Print and shaded views of the part. All mm, measured from the part's lowest x, y and z. A direction names the side the tool comes from. Round coordinates to 2 decimals unless told otherwise and drop trailing zeros. Loops run counter-clockwise (first coordinate to the right, second up) from the corner with the lowest first, then second, coordinate; pieces in that order, holes last. Notation, with made-up numbers: (-33, -14) - (-25, -14) arc R25 ccw to (-25, 2) - close; hole circle Ø11 at (15, 15.25). An arc over 180 degrees is marked (long way). Answer as a JSON object with one key per item and string values.
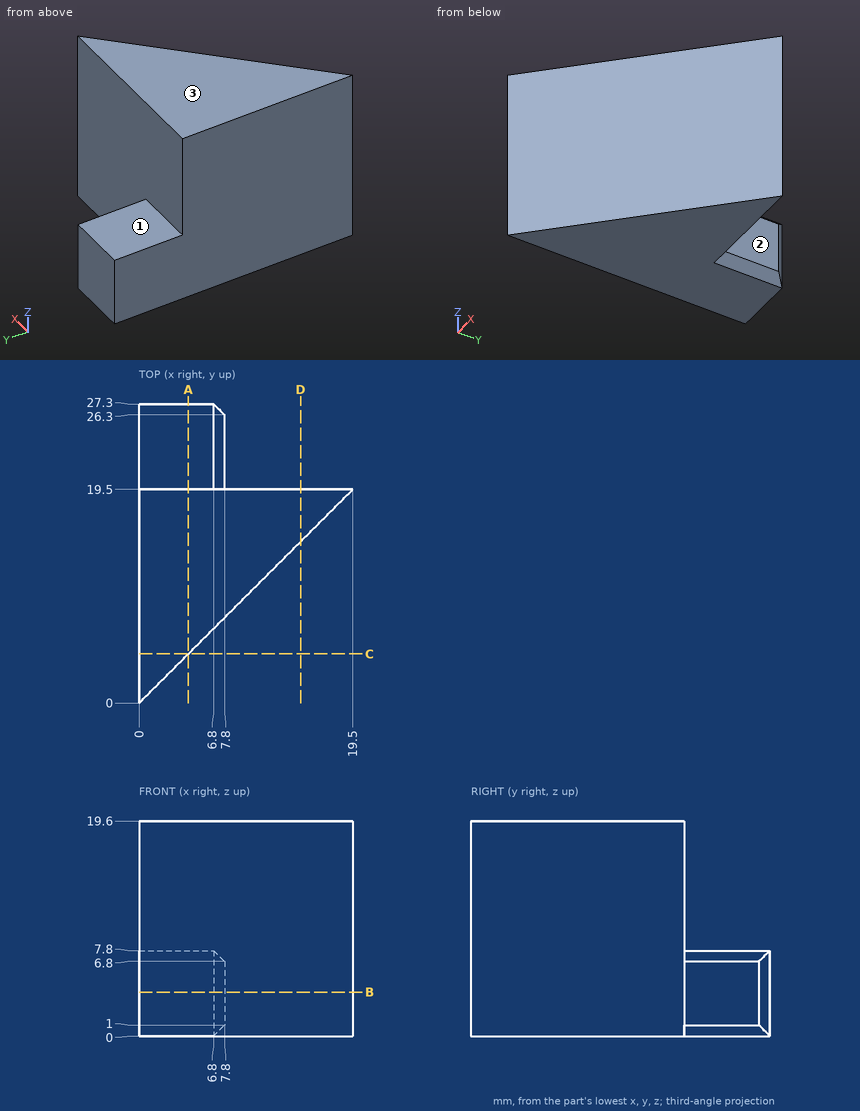
1) Slice it at C-C on y = 4.5. List the corners of the cut face in (x, z).
Values follow:
{"outline": "(0, 0) - (4.5, 0) - (4.5, 19.6) - (0, 19.6) - close"}
2) Slice it at B-B on z = 4. List the corners of the cut face in (x, y), then the cut area to 3 significant figures.
Values follow:
{"outline": "(0, 0) - (19.5, 19.5) - (7.8, 19.5) - (7.8, 26.3) - (6.8, 27.3) - (0, 27.3) - close", "area": "250 mm²"}
3) Slice it at A-A on x = 4.5. List the corners of the cut face in (y, z).
Values follow:
{"outline": "(4.5, 0) - (27.3, 0) - (27.3, 7.8) - (19.5, 7.8) - (19.5, 19.6) - (4.5, 19.6) - close"}
4) Tool access for the marked faces 1, 2 and 3: list every direction of +Z, -Z, +X, -X, +Y, -Y with a clear straight run to the whole face (end or side of a thin tool).
Values follow:
{"face 1": "+Z, +X, -X, +Y", "face 2": "+Z, -Z, +X, +Y", "face 3": "+Z, +X, -X, +Y, -Y"}
5) Probe probe 1 along Z at (x, y) = (5, 25.5); probe 2 along Y at (x, z) = (9, 18.25). List the from-to ranges inside material, lowest first.
Values follow:
{"probe 1": "0 to 7.8", "probe 2": "9 to 19.5"}
6) Drop flat-ended pins along their axis: P1, Ø5, axis at x = 16.5, z = 9, coming from the +Y side; P2, Ø2, axis at y = 23.5, z = 3.5, coming from the +X side; P3, Ø4, axis at y = 4.5, z = 17.5, coming from the +X side. Give the stop position or say it passes through.
Values follow:
{"P1": "y = 19.5", "P2": "x = 7.8", "P3": "x = 6.5"}
7) Slice it at D-D on x = 14.75. List the corners of the cut face in (y, z), then the cut area to 3 significant figures.
Values follow:
{"outline": "(14.75, 0) - (19.5, 0) - (19.5, 19.6) - (14.75, 19.6) - close", "area": "93.1 mm²"}
